from build123d import *

# Parameters (mm, degrees)
SKETCH1_R               = 3.025
BOSS_EXTRUDE1_DEPTH     = 14.1
CUT_EXTRUDE1_DEPTH      = 26.996345897
CUT_EXTRUDE1_DEPTH_BACK = 26.996345897
SKETCH2_W               = 12
SKETCH2_H               = 4.55
SKETCH3_R               = 3.025
CUT_EXTRUDE2_DEPTH      = 27.684452402
CUT_EXTRUDE3_DEPTH      = 10
SKETCH6_R               = 5.05
CUT_EXTRUDE4_DEPTH      = 0.5
SKETCH7_R               = 5.05
CUT_EXTRUDE5_DEPTH      = 0.5
FILLET1_R               = 6
CHAMFER1_SIZE           = 0.2
FILLET2_R               = 0.5


with BuildPart() as part:
    # Sketch1 → Boss-Extrude1 (new body)
    with BuildSketch(Plane(origin=(0, 0, 0), x_dir=(1, 0, 0), z_dir=(0, 1, 0))):
        with BuildLine():
            Line((21, -2.5), (21, 2.5))
            Line((21, 2.5), (5.454356057, 2.5))
            ThreePointArc((5.454356057, 2.5), (-6, 0), (5.454356057, -2.5))
            Line((5.454356057, -2.5), (21, -2.5))
        make_face()
        with Locations(Location((0, 0, 0), (0, 0, 270))):
            Circle(SKETCH1_R, mode=Mode.SUBTRACT)
    extrude(amount=BOSS_EXTRUDE1_DEPTH)

    # Sketch2 → Cut-Extrude1 (cut, two sides: drawn at the far end of the back side and taken through both)
    with BuildSketch(Plane(origin=(0, 0, 0), x_dir=(-1, 0, 0), z_dir=(0, 0, -1)).offset(-CUT_EXTRUDE1_DEPTH_BACK)):
        with Locations((0, 2.275)):
            Rectangle(SKETCH2_W, SKETCH2_H)
        with Locations((0, 11.825)):
            Rectangle(SKETCH2_W, SKETCH2_H)
    extrude(amount=CUT_EXTRUDE1_DEPTH + CUT_EXTRUDE1_DEPTH_BACK, mode=Mode.SUBTRACT)

    # Sketch3 → Cut-Extrude2 (cut, through all)
    with BuildSketch(Plane(origin=(0, 0, -2.5), x_dir=(-1, 0, 0), z_dir=(0, 0, -1))):
        with Locations((-13.5, 7.05)):
            Circle(SKETCH3_R)
    extrude(amount=-CUT_EXTRUDE2_DEPTH, mode=Mode.SUBTRACT)

    # Sketch4 → Cut-Extrude3 (cut)
    with BuildSketch(Plane(origin=(0, 0, -2.5), x_dir=(-1, 0, 0), z_dir=(0, 0, -1))):
        with BuildLine():
            Line((-6, 9.55), (-8.045643943, 9.55))
            ThreePointArc((-8.045643943, 9.55), (-19.5, 7.05), (-8.045643943, 4.55))
            Line((-8.045643943, 4.55), (-6, 4.55))
            Line((-6, 4.55), (-6, 0))
            Line((-6, 0), (-21, 0))
            Line((-21, 0), (-21, 14.1))
            Line((-21, 14.1), (-6, 14.1))
            Line((-6, 14.1), (-6, 9.55))
        make_face()
    extrude(amount=-CUT_EXTRUDE3_DEPTH, mode=Mode.SUBTRACT)

    # Sketch6 → Cut-Extrude4 (cut)
    with BuildSketch(Plane(origin=(0, 9.55, 0), x_dir=(1, 0, 0), z_dir=(0, 1, 0))):
        with Locations(Location((0, 0, 0), (0, 0, 270))):
            Circle(SKETCH6_R)
    extrude(amount=-CUT_EXTRUDE4_DEPTH, mode=Mode.SUBTRACT)

    # Sketch7 → Cut-Extrude5 (cut)
    with BuildSketch(Plane.XY.offset(2.5)):
        with Locations((13.5, 7.05)):
            Circle(SKETCH7_R)
    extrude(amount=-CUT_EXTRUDE5_DEPTH, mode=Mode.SUBTRACT)

    # Fillet1
    fillet1_edges = [part.edges().sort_by_distance(p)[0] for p in [
        (5.454356057, 7.05, 2.5),
    ]]
    fillet(fillet1_edges, radius=FILLET1_R)
    fillet1_2_edges = [part.edges().sort_by_distance(p)[0] for p in [
        (8.045643943, 4.55, 0.007531715),
    ]]
    fillet(fillet1_2_edges, radius=FILLET1_R)
    fillet1_3_edges = [part.edges().sort_by_distance(p)[0] for p in [
        (5.454356057, 7.042468285, -2.5),
    ]]
    fillet(fillet1_3_edges, radius=FILLET1_R)
    fillet1_4_edges = [part.edges().sort_by_distance(p)[0] for p in [
        (8.045643943, 9.55, 0),
    ]]
    fillet(fillet1_4_edges, radius=FILLET1_R)

    # Chamfer1
    chamfer1_edges = [part.edges().sort_by_distance(p)[0] for p in [
        (0, 9.05, -3.025),
        (16.525, 7.05, 2),
        (0, 4.55, -3.025),
        (16.525, 7.05, -2.5),
    ]]
    chamfer(chamfer1_edges, length=CHAMFER1_SIZE)

    # Fillet2
    fillet2_edges = [part.edges().sort_by_distance(p)[0] for p in [
        (-6, 9.55, 0),
        (19.5, 7.05, 2.5),
        (19.5, 7.05, -2.5),
        (-6, 4.55, 0),
        (8.882017401, 10.950236609, -2.5),
        (8.882017401, 10.950236609, 2.5),
        (4.617982599, 4.55, 3.900236609),
        (4.617982599, 9.55, 3.900236609),
        (8.882017401, 3.149763391, -2.5),
        (8.882017401, 3.149763391, 2.5),
        (4.617982599, 4.55, -3.900236609),
        (4.617982599, 9.55, -3.900236609),
        (6.75, 4.298021558, 2.751978442),
        (6.75, 4.298021558, -2.751978442),
        (6.75, 9.801978442, -2.751978442),
        (6.75, 9.801978442, 2.751978442),
    ]]
    fillet(fillet2_edges, radius=FILLET2_R)


solid = part.part
Source: CAD feature listing. Evaluate the final solid. Frame: model axes, mm. A direction names the side the tool comes from. Coordinates: 2 decimals unless noted, no trailing zeros. One line per question, with ' | ' between items.
1) Line query: line 1 along Y through (x, z) = (13.5, 0.1) (3 decimals); line 2 along X through (y, z) = (9.4, 0); line 3 along X through (y, z) = (9.45, 0). Output: solid intervals per line, ascending.
Report:
line 1: y = 1.05 to 4.025, 10.075 to 13.05 | line 2: x = -5.86 to -5.05, 5.05 to 11.6, 15.4 to 19.02 | line 3: x = -5.8 to -5.05, 5.05 to 11.66, 15.34 to 19
2) Pull-direction query (Y, two-part tool) for faces 5 (the face through (18.165, 5.116, 2.254)), 6 (the face through (0.909, 6.771, 2.885)), 7 (the face through (-1.1, 9.05, 3.3)), 8 (the face through (15.73, 9.094, -0.279)); classes: released by +Y, released by -Y, zero draft, split by the parting line, or undercut.
Report:
face 5: undercut | face 6: zero draft | face 7: released by +Y | face 8: undercut
3) First-contact query: P1, Ø1, axis at x = 13, z = -2.5, coming from the -Y side; P2, Ø4, axis at x = -2, z = 0.5, coming from the -Y side; P3, Ø5, axis at x = 0, z = 0, coming from the +Y side (3 decimals); P4, Ø2, axis at y = 7.5, z = -4, coming from the -X side. Flat tips, straight axial feed; report the tip coordinate or a pass-through.
Report:
P1: stops at y = 1.06 | P2: stops at y = 4.55 | P3: passes through | P4: stops at x = -5.2
4) Section A-A, the plane y = 7.05. Give the number of separate pieces and of enclosed holes in the cut face, then the cut area to 3 significant figures.
Report:
separate pieces: 2 | enclosed holes: 1 | area: 122 mm²
5) Set-up query: faces 1 (the face through (-3, 4.55, -2)), 2 (the face through (17, 11, 2.5)), 3 (the face through (16.1, 9.4, -2.5)), 4 (the face through (17, 7, 2)). Return all of +Z, -Z, +X, -X, +Y, -Y with unobstructed straight access to the full face (end or side cutting, diameter ignored); none if empty.
Report:
face 1: +Z, -Z, -X, -Y | face 2: +Z, +X, +Y, -Y | face 3: -Z, +X, +Y, -Y | face 4: +Z
